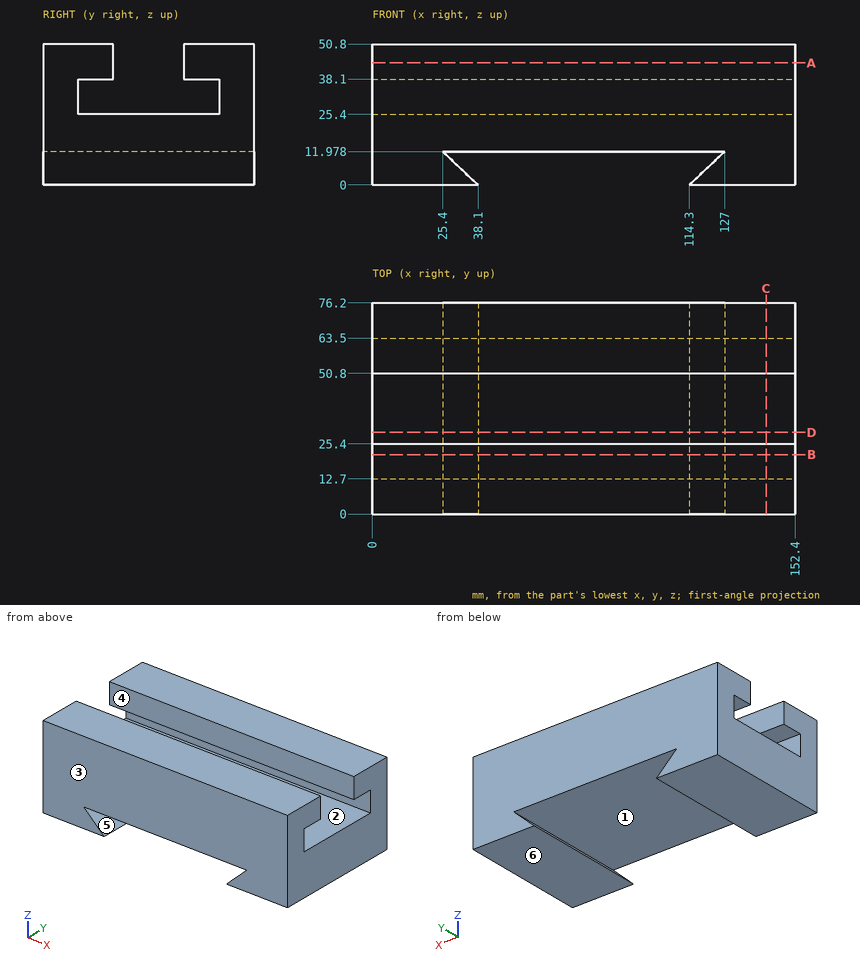
Could you check a few things on this drawing? It's one solid part, dimensions in mm from its lowest x, y, z. A direction names the side the tool comes from. Coordinates: 2 decimals unless noted, no trailing zeros. Order: outer loops, then holes, each group sorted by start corner. A loop starts at its lowest first (then second) coordinate and runs counter-clockwise, first axis right, second up.
1) We'd pull the mould along Y, two halves only. Please class the marked faces 1, 2 and 3: +Y half, -Y half, draft (parallel to the pull), parting line (faces both ways), or undercut.
2) Imagine slicing it at B-B on y = 21.5. List the corners of the cut face in (x, z) for me, and give its area (3 significant figures).
3) Imagine slicing it at A-A on z = 44. List the corners of the cut face in (x, y) for me, and give its area (3 significant figures).
4) Which directions (+Z, -Z, +X, -X, +Y, -Y) give clear straight access to the entire face, cutting with the end or side of a thin tool? Please do the marked faces 4, 5 and 6.
5) Imagine slicing it at D-D on y = 29.5. List the corners of the cut face in (x, z) for me.
6) I need wall thicknesses on line 1 (Z direction, x = 20, y = 54.5); line 2 (Z direction, x = 90.5, y = 15); line 3 (Y direction, x = 54, z = 29). Which ranges of each line are inside material? Lowest first, please.
7) Will these pins go through, and if not, where does the flat tip stop? pin 1 (8 mm diameter, centred on x = 130.5, y = 30.5, fed in from +Z); pin 2 (14 mm diameter, centred on x = 49, y = 20, fed in from -Z).
8) Imagine slicing it at C-C on x = 142. List the corners of the cut face in (y, z) for me.
Response values:
1. face 1: draft
1. face 2: undercut
1. face 3: -Y half
2. outline: (0, 0) - (38.1, 0) - (25.4, 11.98) - (127, 11.98) - (114.3, 0) - (152.4, 0) - (152.4, 25.4) - (0, 25.4) - close; (0, 38.1) - (152.4, 38.1) - (152.4, 50.8) - (0, 50.8) - close
2. area: 4,740 mm2
3. outline: (0, 0) - (152.4, 0) - (152.4, 25.4) - (0, 25.4) - close; (0, 50.8) - (152.4, 50.8) - (152.4, 76.2) - (0, 76.2) - close
3. area: 7,740 mm2
4. face 4: +Z, +X, -X
4. face 5: +Y, -Y
4. face 6: -Z, +X, -X, +Y, -Y
5. outline: (0, 0) - (38.1, 0) - (25.4, 11.98) - (127, 11.98) - (114.3, 0) - (152.4, 0) - (152.4, 25.4) - (0, 25.4) - close
6. line 1: z = 0 to 25.4, 38.1 to 50.8
6. line 2: z = 11.98 to 25.4, 38.1 to 50.8
6. line 3: y = 0 to 12.7, 63.5 to 76.2
7. pin 1: stops at z = 25.4
7. pin 2: stops at z = 11.98
8. outline: (0, 0) - (76.2, 0) - (76.2, 50.8) - (50.8, 50.8) - (50.8, 38.1) - (63.5, 38.1) - (63.5, 25.4) - (12.7, 25.4) - (12.7, 38.1) - (25.4, 38.1) - (25.4, 50.8) - (0, 50.8) - close
